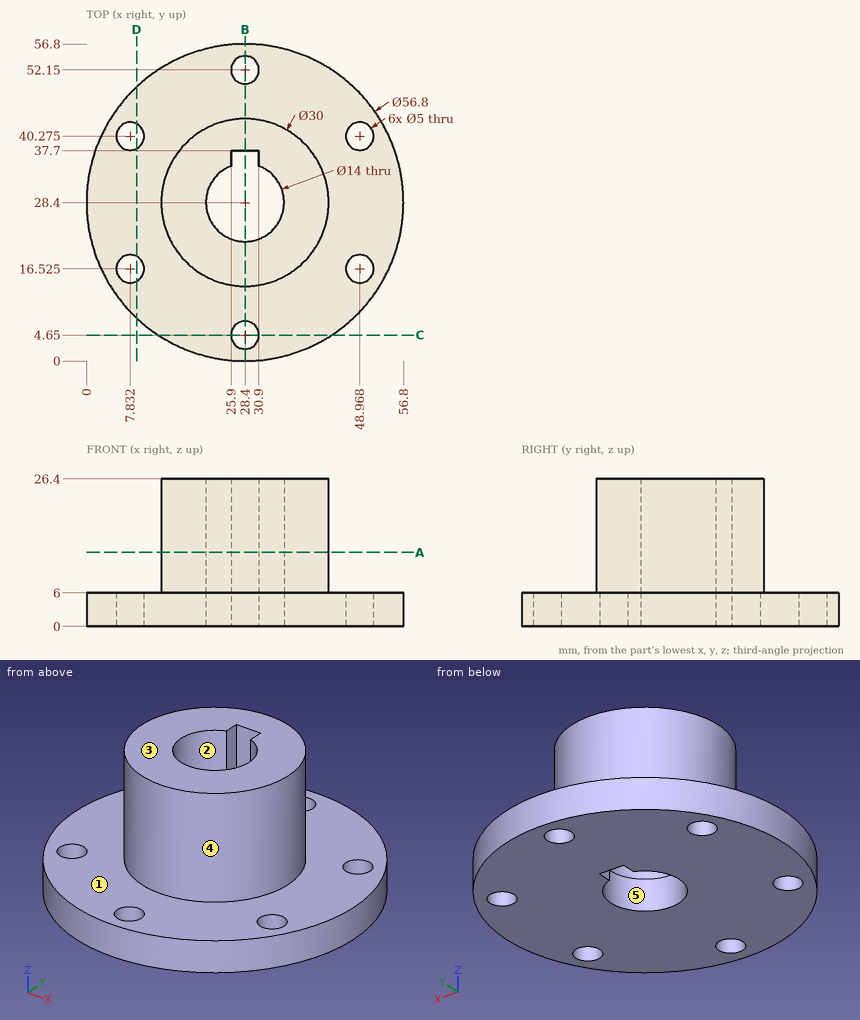
Source: three-view drawing plus pictorial views. Frame: mm from the lowest corner of the part. A direction names the side the tool comes from. Round coordinates to 2 decimals unless told otherwise and drop trailing zeros. Loops run counter-clockwise (first coordinate to the right, second up) from the corner with the lowest first, then second, coordinate; pieces in that order, holes last.
Q1. Access query for the marked faces 1 and 2. Directions: +Z, -Z, +X, -X, +Y, -Y. A direction counts if a zero-diameter tool reaches every point of the face in a straight line with its end or side. Return the directions, or none.
Q2. Section B-B on x = 28.4. Return loops of the section in (y, z).
Q3. Section A-A on z = 13.25. Return loops of the section in (x, y).
Q4. Material intervals for L1, parallel to Y at x = 28.4, z = 4; L2, parallel to X at y = 38.5, z = 4.75; L3, parallel to X at y = 28, z = 10, sorted ascending.
Q5. Pull-direction query (Y, two-part tool) for the marked faces 3, 4 and 5; classes: released by +Y, released by -Y, zero draft, split by the parting line, or undercut.
Q6. Pin query (flat end, axial travel): P1, Ø3, axis at x = 28.4, y = 4.65, coming from the -Z side; P2, Ø5, axis at y = 37.5, z = 15.5, coming from the -X side; P3, Ø6, axis at y = 9, z = 4.5, coming from the +X side; P4, Ø2.5, axis at x = 27.5, z = 12.5, coming from the -Y side. Return the tip coordinate at first contact, or that it passes through.
Q7. Section D-D on x = 9. Return loops of the section in (y, z).
Q8. Section C-C on y = 4.65. Return loops of the section in (x, z), plus the area to 3 significant figures.
Evaluation:
1. face 1: +Z
1. face 2: +Z, -Z
2. outline: (0, 0) - (2.15, 0) - (2.15, 6) - (0, 6) - close; (7.15, 0) - (21.4, 0) - (21.4, 26.4) - (13.4, 26.4) - (13.4, 6) - (7.15, 6) - close; (37.7, 0) - (49.65, 0) - (49.65, 6) - (43.4, 6) - (43.4, 26.4) - (37.7, 26.4) - close; (54.65, 0) - (56.8, 0) - (56.8, 6) - (54.65, 6) - close
3. outline: circle Ø30 at (28.4, 28.4); hole (25.9, 34.94) arc R7 ccw (long way) to (30.9, 34.94) - (30.9, 37.7) - (25.9, 37.7) - close
4. L1: y = 0 to 2.15, 7.15 to 21.4, 37.7 to 49.65, 54.65 to 56.8
4. L2: x = 1.86 to 6.07, 9.59 to 47.21, 50.73 to 54.94
4. L3: x = 13.41 to 21.41, 35.39 to 43.39
5. face 3: zero draft
5. face 4: split by the parting line
5. face 5: undercut
6. P1: passes through
6. P2: stops at x = 14.93
6. P3: stops at x = 51.59
6. P4: stops at y = 13.4
7. outline: (7.66, 0) - (14.31, 0) - (14.31, 6) - (7.66, 6) - close; (18.74, 0) - (38.06, 0) - (38.06, 6) - (18.74, 6) - close; (42.49, 0) - (49.14, 0) - (49.14, 6) - (42.49, 6) - close
8. outline: (12.83, 0) - (25.9, 0) - (25.9, 6) - (12.83, 6) - close; (30.9, 0) - (43.97, 0) - (43.97, 6) - (30.9, 6) - close
8. area: 157 mm2
